from build123d import *

# Parameters (mm, degrees)
SKETCH1_W            = 85.48
SKETCH1_H            = 52.4
BOSS_EXTRUDE1_DEPTH  = 2
BOSS_EXTRUDE2_DEPTH  = 2
SKETCH7_W            = 3
SKETCH7_H            = 5
SKETCH7_W_2          = 0.4
CUT_EXTRUDE2_DEPTH   = 55.775428798
FILLET4_R            = 1
FILLET4_OF_MIRROR2_R = 1
SKETCH8_W            = 85.48
SKETCH8_H            = 1
BOSS_EXTRUDE4_DEPTH  = 2
FILLET5_START        = -42.74
FILLET5_DEPTH        = 85.48
FILLET5_START_2      = -19.34
FILLET5_2_DEPTH      = 38.68
FILLET5_3_DEPTH      = 16.6
FILLET5_START_3      = 26.14
FILLET5_4_DEPTH      = 16.6
FILLET6_R            = 0.5


with BuildPart() as part:
    # Sketch1 → Boss-Extrude1 (new body)
    with BuildSketch(Plane.XY):
        Rectangle(SKETCH1_W, SKETCH1_H)
    extrude(amount=BOSS_EXTRUDE1_DEPTH)

    # Sketch2 → Boss-Extrude2 (add)
    with BuildSketch(Plane(origin=(0, 0, 0), x_dir=(-1, 0, 0), z_dir=(0, 0, -1))):
        Polygon((-27.24, 27.7), (-25.74, 27.7), (-25.74, 26.2), (-24.24, 26.2), (-24.24, 29.2), (-25.74, 29.2), align=None)
        Polygon((-19.74, 29.2), (-21.24, 29.2), (-21.24, 26.2), (-19.74, 26.2), (-19.74, 27.7), (-18.24, 27.7), align=None)
        Polygon((-25.773724333, -26.2), (-25.773724333, -32.7), (-27.273724333, -32.7), (-25.773724333, -34.2), (-24.273724333, -34.2), (-24.273724333, -26.2), align=None)
        Polygon((-21.273724333, -26.2), (-21.273724333, -34.2), (-19.773724333, -34.2), (-18.273724333, -32.7), (-19.773724333, -32.7), (-19.773724333, -26.2), align=None)
    boss_extrude2 = extrude(amount=-BOSS_EXTRUDE2_DEPTH)

    # Sketch7 → Cut-Extrude2 (cut, through all)
    with BuildSketch(Plane.XY.offset(2)):
        with Locations((22.74, 23.7)):
            Rectangle(SKETCH7_W, SKETCH7_H)
        with Locations((19.54, 23.7)):
            Rectangle(SKETCH7_W_2, SKETCH7_H)
        with Locations((25.94, 23.7)):
            Rectangle(SKETCH7_W_2, SKETCH7_H)
    cut_extrude2 = extrude(amount=-CUT_EXTRUDE2_DEPTH, mode=Mode.SUBTRACT)

    # Fillet4
    fillet4_edges = [part.edges().sort_by_distance(p)[0] for p in [
        (19.34, 26.2, 1),
        (21.24, 21.2, 1),
        (24.24, 21.2, 1),
        (24.273724333, -26.2, 1),
        (21.273724333, -26.2, 1),
        (26.14, 26.2, 1),
    ]]
    fillet(fillet4_edges, radius=FILLET4_R)

    # Mirror2: Boss-Extrude2, Cut-Extrude2 across plane
    add(boss_extrude2.mirror(Plane(origin=(0, 0, 0), x_dir=(0, 0, 1), z_dir=(1, 0, 0))))
    add(cut_extrude2.mirror(Plane(origin=(0, 0, 0), x_dir=(0, 0, 1), z_dir=(1, 0, 0))), mode=Mode.SUBTRACT)

    # Fillet4 of Mirror2
    fillet4_of_mirror2_edges = [part.edges().sort_by_distance(p)[0] for p in [
        (-19.34, 26.2, 1),
        (-21.24, 21.2, 1),
        (-24.24, 21.2, 1),
        (-24.273724333, -26.2, 1),
        (-21.273724333, -26.2, 1),
        (-26.14, 26.2, 1),
    ]]
    fillet(fillet4_of_mirror2_edges, radius=FILLET4_OF_MIRROR2_R)

    # Sketch8 → Boss-Extrude4 (add)
    with BuildSketch(Plane.XY.offset(2)):
        with BuildLine():
            Line((-42.74, 26.2), (-42.74, 25.2))
            Line((-42.74, 25.2), (-26.14, 25.2))
            ThreePointArc((-26.14, 25.2), (-26.432893219, 25.907106781), (-27.14, 26.2))
            Line((-27.14, 26.2), (-42.74, 26.2))
        make_face()
        with BuildLine():
            ThreePointArc((-18.34, 26.2), (-19.047106781, 25.907106781), (-19.34, 25.2))
            Line((-19.34, 25.2), (19.34, 25.2))
            ThreePointArc((19.34, 25.2), (19.047106781, 25.907106781), (18.34, 26.2))
            Line((18.34, 26.2), (-18.34, 26.2))
        make_face()
        with BuildLine():
            Line((26.14, 25.2), (42.74, 25.2))
            Line((42.74, 25.2), (42.74, 26.2))
            Line((42.74, 26.2), (27.14, 26.2))
            ThreePointArc((27.14, 26.2), (26.432893219, 25.907106781), (26.14, 25.2))
        make_face()
        with Locations((0, -25.7)):
            Rectangle(SKETCH8_W, SKETCH8_H)
    extrude(amount=BOSS_EXTRUDE4_DEPTH)

    # Fillet5: read off the stored shape, not the designer's step
    # Fillet5 outline → Fillet5 (add)
    with BuildSketch(Plane.YZ.offset(FILLET5_START)):
        with BuildLine():
            Line((-25.2, 2), (-21.2, 2))
            add(Edge.make_bspline(
                [(-21.2, 2), (-23.7, 2), (-25.2, 4)],
                knots=[0, 0, 0, 1, 1, 1], degree=2, weights=[1, 0.894427191, 1]))
            Line((-25.2, 4), (-25.2, 2))
        make_face()
    extrude(amount=FILLET5_DEPTH)

    # Fillet5 2 outline → Fillet5 2 (add)
    with BuildSketch(Plane.YZ.offset(FILLET5_START_2)):
        with BuildLine():
            add(Edge.make_bspline(
                [(25.2, 4), (23.7, 2), (21.2, 2)],
                knots=[0, 0, 0, 1, 1, 1], degree=2, weights=[1, 0.894427191, 1]))
            Line((21.2, 2), (25.2, 2))
            Line((25.2, 2), (25.2, 4))
        make_face()
    extrude(amount=FILLET5_2_DEPTH)

    # Fillet5 3 outline → Fillet5 3 (add)
    with BuildSketch(Plane.YZ.offset(FILLET5_START)):
        with BuildLine():
            add(Edge.make_bspline(
                [(25.2, 4), (23.7, 2), (21.2, 2)],
                knots=[0, 0, 0, 1, 1, 1], degree=2, weights=[1, 0.894427191, 1]))
            Line((21.2, 2), (25.2, 2))
            Line((25.2, 2), (25.2, 4))
        make_face()
    extrude(amount=FILLET5_3_DEPTH)

    # Fillet5 4 outline → Fillet5 4 (add)
    with BuildSketch(Plane.YZ.offset(FILLET5_START_3)):
        with BuildLine():
            add(Edge.make_bspline(
                [(25.2, 4), (23.7, 2), (21.2, 2)],
                knots=[0, 0, 0, 1, 1, 1], degree=2, weights=[1, 0.894427191, 1]))
            Line((21.2, 2), (25.2, 2))
            Line((25.2, 2), (25.2, 4))
        make_face()
    extrude(amount=FILLET5_4_DEPTH)

    # Fillet6
    fillet6_edges = [part.edges().sort_by_distance(p)[0] for p in [
        (-42.74, 26.2, 2),
        (42.74, 26.2, 2),
        (42.74, -26.2, 2),
        (-42.74, -26.2, 2),
    ]]
    fillet(fillet6_edges, radius=FILLET6_R)


solid = part.part
Geometry check sheet. Reference: the model listing, model coordinates, mm. A direction names the side the tool comes from. Round coordinates to 2 decimals unless told otherwise and drop trailing zeros. Write each loop counter-clockwise with the first axis right and the second up, starting at its lowest first coordinate (ties: lowest second). Pieces come first, ordered by that corner, then holes. Notation, with made-up numbers: (78, -13.75) -> (92, -13.75) arc R27 ccw to (92, 19.25) -> close; hole circle Ø8 at (-22.5, 62.5). An arc over 180 degrees is marked (long way). One line per item, written item: value. Start each with the question number.
(1) Access from +Z, -Z, +X, -X, +Y, -Y to the whole of each face (thin tool, end or side, straight path). Record for faces 4 (the flat face through (25, -30, 2)), 5 (the flat face through (19.34, 23, 1)), 6 (the flat face through (24.274, -31, 1)), 7 (the flat face through (24.24, 26, 1)), 8 (the flat face through (42.74, 0, 1)).
(2) Go/stop test with flat-tipped pins: pin 1 Ø0.8 at (x, z) = (-19, 1) entering from -Y; pin 2 Ø0.8 at (x, z) = (23, 1) entering from +Y; pin 3 Ø1.2 at (x, z) = (-38.5, 2.5) entering from +Y. Record where each tip stops, or that it passes through.
(3) Scan lines: line 1 (X direction, y = -28.5, z = 1.1); line 2 (Z direction, x = -32.5, y = -6); line 3 (Y direction, x = -8.5, z = 3.55). Record each from-to range of solid material in increasing order. Write a range as [from, to].
(4) Cross-section at B-B, the plane z = 3.3. Give the number of separate pieces and of enclosed holes in the cut face, and give its area (3 significant figures).
(5) Draft check along Y on faces 1 (the flat face through (-25, -30, 2)), 2 (the flat face through (-26.14, 23, 1)), 3 (the flat face through (26.14, 23, 1)). Enter one of: +Y half, -Y half, draft (parallel to the pull), parting line (faces both ways), or undercut.
(6) Cross-section at A-A, the plane y = 3.5. Record the cut outline in (x, z).
Answer:
1. face 4: +Z, +X, -X, -Y
1. face 5: +Z, -Z
1. face 6: +Z, -Z, -Y
1. face 7: +Z, -Z, +Y
1. face 8: +Z, -Z, +X, +Y, -Y
2. pin 1: y = -33.83
2. pin 2: y = 21.21
2. pin 3: y = 26.2
3. line 1: [-25.77, -24.27], [-21.27, -19.77], [19.77, 21.27], [24.27, 25.77]
3. line 2: [0, 2]
3. line 3: [-26.2, -24.82], [24.82, 26.2]
4. separate pieces: 4
4. enclosed holes: 0
4. area: 257 mm²
5. face 1: draft
5. face 2: undercut
5. face 3: undercut
6. outline: (-42.74, 0) -> (42.74, 0) -> (42.74, 2) -> (-42.74, 2) -> close
